Read the model definition and answer for the solid it produces. Units are mm, in the model's axes. Give positions to 0.01 mm unless a question says otherwise; leave off trailing zeros. Order: outer loops, then holes, each group sorted by start corner. A loop starts at its lowest first (then second) coordinate and runs counter-clockwise, first axis right, second up. Notation, with made-up numbers: (66.25, 8.25) - (116.25, 8.25) arc R13 ccw to (116.25, 14.25) - close; hole circle Ø7 at (-35.5, 11). An arc over 180 degrees is marked (long way). Write item = value, one per line.
Autodesk Inventor part; units mm, degrees
ref_plane "YZ Plane" through (0, 0, 0) normal (1, 0, 0) x (0, 1, 0)
ref_plane "XZ Plane" through (0, 0, 0) normal (0, 1, 0) x (-1, 0, 0)
ref_plane "XY Plane" through (0, 0, 0) normal (0, 0, 1) x (1, 0, 0)
sketch "Esboço1" plane through (0, 0, 0) normal (1, 0, 0) x (0, 1, 0)
  line L0 (-504, 129) -> (504, 129)
  line L1 (504, 129) -> (504, -129)
  line L2 (504, -129) -> (-504, -129)
  line L3 (-504, -129) -> (-504, 129)
  line L4 (-504, 129) -> (504, -129) construction
  line L5 (504, 129) -> (-504, -129) construction
  point P0 (0, 0)
  dimension "d0" = 1008
  dimension "d1" = 258
extrude "Extrusão1" add sketch "Esboço1" along normal mid plane 4
sketch "Esboço2" plane through (2, 0, 0) normal (1, 0, 0) x (0, 0, -1)
  line L0 (-133, 378) -> (-125, 378)
  line L1 (-125, 378) -> (-125, 126)
  line L2 (-125, 126) -> (-133, 126)
  line L3 (-133, 126) -> (-133, 378)
  line L4 (-129, 504) -> (-129, -504)
  line L5 (-133, 378) -> (-125, 126) construction
  line L6 (-125, 378) -> (-133, 126) construction
  line L7 (129, 504) -> (-129, 504)
  line L8 (-133, -126) -> (-125, -126)
  line L9 (-125, -126) -> (-125, -378)
  line L10 (-125, -378) -> (-133, -378)
  line L11 (-133, -378) -> (-133, -126)
  line L12 (-133, -126) -> (-125, -378) construction
  line L13 (-125, -126) -> (-133, -378) construction
  line L14 (-129, -504) -> (129, -504)
  line L15 (125, 378) -> (133, 378)
  line L16 (133, 378) -> (133, 126)
  line L17 (133, 126) -> (125, 126)
  line L18 (125, 126) -> (125, 378)
  line L19 (129, -504) -> (129, 504)
  line L20 (125, 378) -> (133, 126) construction
  line L21 (133, 378) -> (125, 126) construction
  line L22 (125, -126) -> (133, -126)
  line L23 (133, -126) -> (133, -378)
  line L24 (133, -378) -> (125, -378)
  line L25 (125, -378) -> (125, -126)
  line L26 (125, -126) -> (133, -378) construction
  line L27 (133, -126) -> (125, -378) construction
  point P0 (0, 0)
  point P1 (-129, 252)
  point P2 (-129, -252)
  point P3 (129, 252)
  point P4 (129, -252)
  dimension "d4" = 8
  dimension "d5" = 252
  dimension "d6" = 126
  dimension "d7" = 8
  dimension "d8" = 252
  dimension "d9" = 252
  dimension "d10" = 126
  dimension "d11" = 126
  dimension "d12" = 252
  dimension "d13" = 8
  dimension "d14" = 252
  dimension "d15" = 8
  dimension "d16" = 252
  dimension "d17" = 126
extrude "Extrusão2" cut sketch "Esboço2" along normal through all both and the other way through all contours L0 L4 L2 L3 | L0 L1 L2 L4 | L8 L9 L10 L4 | L4 L10 L11 L8 | L19 L17 L18 L15 | L15 L16 L17 L19 | L22 L23 L24 L19 | L19 L24 L25 L22
sketch "Esboço3" plane through (2, 0, 0) normal (1, 0, 0) x (0, 0, -1)
  line L0 (-41.5, 500) -> (41.5, 500)
  line L1 (41.5, 500) -> (41.5, 508)
  line L2 (41.5, 508) -> (-41.5, 508)
  line L3 (-41.5, 508) -> (-41.5, 500)
  line L4 (129, 504) -> (-129, 504)
  line L5 (-41.5, 500) -> (41.5, 508) construction
  line L6 (41.5, 500) -> (-41.5, 508) construction
  line L7 (-41.5, -500) -> (41.5, -500)
  line L8 (41.5, -500) -> (41.5, -508)
  line L9 (41.5, -508) -> (-41.5, -508)
  line L10 (-41.5, -508) -> (-41.5, -500)
  line L11 (-129, -504) -> (129, -504)
  line L12 (-41.5, -500) -> (41.5, -508) construction
  line L13 (41.5, -500) -> (-41.5, -508) construction
  point P0 (0, 0)
  point P1 (0, 504)
  point P2 (0, -504)
  dimension "d20" = 83
  dimension "d21" = 8
  dimension "d22" = 83
  dimension "d23" = 8
extrude "Extrusão3" cut sketch "Esboço3" along normal through all both and the other way through all
sketch "Esboço5" plane through (2, 0, 0) normal (1, 0, 0) x (0, 0, -1)
  line L0 (41.5, 500) -> (-41.5, 500)
  line L1 (0, 400) -> (-80, 400)
  line L2 (-125, 378) -> (-125, 126)
  line L3 (0, 400) -> (80, 400)
  line L4 (-80, 400) -> (-80, 166.6667)
  line L5 (-80, 166.6667) -> (80, 166.6667)
  line L6 (80, 166.6667) -> (80, 400)
  point P0 (0, 0)
  dimension "d39" = 80
  dimension "d40" = 80
  dimension "d41" = 233.3333
  dimension "d67" = 45
extrude "Extrusão5" cut sketch "Esboço5" against normal through all
pattern_linear "Padrão retangular2" count 3 spacing 283.3333 along (0, -1, 0) of "Extrusão5"
sketch "Esboço6" plane through (2, 0, 0) normal (1, 0, 0) x (0, 0, -1)
  line L0 (-80, -166.6667) -> (80, -166.6667)
  line L1 (80, -116.6667) -> (-80, -116.6667)
  line L2 (-80, -116.6667) -> (-30, -116.6667)
  line L3 (80, -116.6667) -> (30, -116.6667)
  line L4 (30, -116.6667) -> (-30, -116.6667)
  line L5 (-35, -129.1667) -> (35, -129.1667)
  line L6 (35, -129.1667) -> (35, -154.1667)
  line L7 (35, -154.1667) -> (-35, -154.1667)
  line L8 (-35, -129.1667) -> (-35, -154.1667)
  line L9 (-125, -126) -> (-125, -378)
  point P0 (0, 0)
  point P1 (-35, -141.6667)
  dimension "d51" = 25
  dimension "d68" = 90
  dimension "d69" = 12.5
  dimension "d70" = 70
extrude "Extrusão6" cut sketch "Esboço6" against normal through all
pattern_linear "Padrão retangular3" count 3 spacing 283.3333 along (0, 1, 0) of "Extrusão6"
sketch "Esboço7" plane through (2, 0, 0) normal (1, 0, 0) x (0, 0, -1)
  line L0 (-80, -400) -> (-80, -166.6667)
  line L1 (-125, -126) -> (-125, -378)
  line L2 (-80, 166.6667) -> (-80, 400)
  line L3 (-107.5, 280.8333) -> (-102.5, 280.8333)
  line L4 (-102.5, 280.8333) -> (-102.5, 285.8333)
  line L5 (-102.5, 285.8333) -> (-107.5, 285.8333)
  line L6 (-107.5, 285.8333) -> (-107.5, 280.8333)
  line L7 (-107.5, 280.8333) -> (-102.5, 285.8333) construction
  line L8 (-102.5, 280.8333) -> (-107.5, 285.8333) construction
  point P0 (0, 0)
  dimension "d60" = 5
  dimension "d61" = 5
extrude "Extrusão7" cut sketch "Esboço7" against normal through all
pattern_linear "Padrão retangular4" count 3 spacing 283.3333 along (0, -1, 0) of "Extrusão7"
properties part number "PAREDE FRONTAL"
1. Straight lines are drawn through the part: L1, parallel to Y at x = 1.55, z = 49; L2, parallel to Y at x = -1.1, z = 40; L3, parallel to Z at x = 0.55, y = -202. For each, find the intervals that lie inside material, in ascending order. Write a range as [from, to].
Recorded:
L1 = [-504, -400], [-166.67, -116.67], [116.67, 166.67], [400, 504]
L2 = [-500, -400], [-166.67, -116.67], [116.67, 166.67], [400, 500]
L3 = [-125, -80], [80, 125]
2. Determine the mould class of faces 1 (the face through (-2, -7, 88)), 2 (the face through (2, -7, 88)) for opening direction X: +X half, -X half, draft (parallel to the pull), parting line (faces both ways), or undercut.
Recorded:
face_1 = -X half
face_2 = +X half
3. Section C-C (z = 1) is taken. Determine the outline of the cut face in (x, y).
Recorded:
outline = (-2, -500) - (2, -500) - (2, -400) - (-2, -400) - close; (-2, -166.67) - (2, -166.67) - (2, -154.17) - (-2, -154.17) - close; (-2, -129.17) - (2, -129.17) - (2, -116.67) - (-2, -116.67) - close; (-2, 116.67) - (2, 116.67) - (2, 129.17) - (-2, 129.17) - close; (-2, 154.17) - (2, 154.17) - (2, 166.67) - (-2, 166.67) - close; (-2, 400) - (2, 400) - (2, 412.5) - (-2, 412.5) - close; (-2, 437.5) - (2, 437.5) - (2, 500) - (-2, 500) - close
4. Section B-B (y = -98.5) is taken. Determine the outline of the cut face in (x, z), and give its area (3 significant figures).
Recorded:
outline = (-2, -129) - (2, -129) - (2, -80) - (-2, -80) - close; (-2, 80) - (2, 80) - (2, 129) - (-2, 129) - close
area = 392 mm^2
5. Flat-ended cylindrical pins translate along their axes: pin 1 (2 mm diameter, centred on x = 0.5, z = -17.5, fed in from +Y); pin 2 (2 mm diameter, centred on x = 1, y = 283.5, fed in from +Z); pin 3 (1.2 mm diameter, centred on x = -0.5, z = -20.5, fed in from -Y). Find the tip coordinate at first contact, or state that the pin passes through.
Recorded:
pin_1 = 500
pin_2 = 125
pin_3 = -500
6. Section A-A (z = 62) is taken. Determine the outline of the cut face in (x, y), and give its area (3 significant figures).
Recorded:
outline = (-2, -504) - (2, -504) - (2, -400) - (-2, -400) - close; (-2, -166.67) - (2, -166.67) - (2, -116.67) - (-2, -116.67) - close; (-2, 116.67) - (2, 116.67) - (2, 166.67) - (-2, 166.67) - close; (-2, 400) - (2, 400) - (2, 504) - (-2, 504) - close
area = 1,230 mm^2
7. Section D-D (x = -0.6) is taken. Count the separate pieces of the cut face and the enclosed holes in it, and give its area (3 significant figures).
Recorded:
separate_pieces = 1
enclosed_holes = 9
area = 138,000 mm^2
